Drawing for the job (mm, zero at the part's lowest x, y, z). Coordinates: 2 decimals unless noted, no trailing zeros. Loops run counter-clockwise (first coordinate to the right, second up) from the corner with the lowest first, then second, coordinate; pieces in that order, holes last. Notation, with made-up numbers: (19.25, -7.75) - (35.25, -7.75) arc R23 ccw to (35.25, 22.25) - close; hole circle Ø6 at (-13, 59). An arc over 180 degrees is marked (long way). One line per item, written item: value.
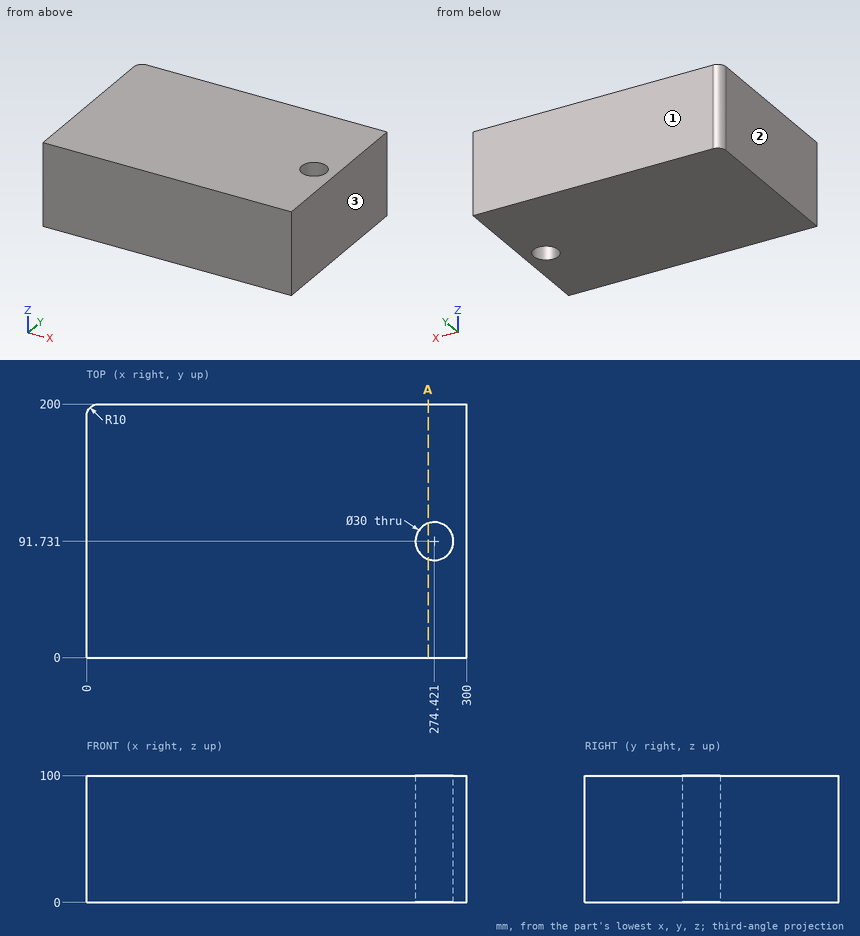
Item 1: Pull direction X, two halves, no side cores. Call the marked faces 1, 2 and 3: released by +X, released by -X, zero draft, split by the parting line, or undercut.
Check result:
face 1: zero draft
face 2: released by -X
face 3: released by +X
Item 2: Cut at A-A, the plane x = 269.5. Write the cut outline in (y, z), then the cut area to 3 significant figures.
Check result:
outline: (0, 0) - (77.56, 0) - (77.56, 100) - (0, 100) - close; (105.9, 0) - (200, 0) - (200, 100) - (105.9, 100) - close
area: 17,200 mm^2
Item 3: Probe probe 1 along X at (y, z) = (83, 26) (1 decimal); probe 2 along Y at (x, z) = (282.5, 59); probe 3 along Y at (x, z) = (285, 44.5) (1 decimal). List the from-to ranges inside material, lowest first. Write a range as from..to.
Check result:
probe 1: x = 0..262.2, 286.6..300
probe 2: y = 0..79.09, 104.37..200
probe 3: y = 0..81.1, 102.4..200
